Design review of the part built by this model. Coordinates are the model's own, in mm. A direction names the side the tool comes from. Give positions to 0.01 mm unless a question says otherwise; leave off trailing zeros. Write each loop counter-clockwise with the first axis right and the second up, starting at its lowest first coordinate (ties: lowest second). Pieces come first, ordered by that corner, then holes. Notation, with made-up numbers: M 22,54 L 62,54 A13 cw 62,65 Z; hole C 7,-2 d10. An arc over 180 degrees is marked long. Write each question's results on one line, items separated by ' | '. Start each with the question number.
from build123d import *

# Parameters (mm, degrees)
F1_DEPTH = 2
F3_DEPTH = 20
F5_DEPTH = 2


with BuildPart() as f1:
    # F0 (on Top) → F1 (new body)
    with BuildSketch(Plane.XY):
        with BuildLine():
            ThreePointArc((5.3033008589, 5.3033008589), (-6.9290964938, -2.8701257427), (7.5, 0))
            Line((7.5, 0), (5, 0))
            ThreePointArc((5, 0), (-4.6193976626, -1.9134171618), (3.5355339059, 3.5355339059))
            Line((3.5355339059, 3.5355339059), (5.3033008589, 5.3033008589))
        make_face()
        with BuildLine():
            ThreePointArc((3.5355339059, 3.5355339059), (-4.6193976626, -1.9134171618), (5, 0))
            Line((5, 0), (4.6, 0))
            ThreePointArc((4.6, 0), (-4.2498458496, -1.7603437889), (3.2526911935, 3.2526911935))
            Line((3.2526911935, 3.2526911935), (3.5355339059, 3.5355339059))
        make_face()
    extrude(amount=F1_DEPTH)

    # F2 (on face) → F3 (join)
    with BuildSketch(Plane.XY.offset(2)):
        with BuildLine():
            Line((7.5, 0), (5, 0))
            ThreePointArc((5, 0), (-4.6193976626, -1.9134171618), (3.5355339059, 3.5355339059))
            Line((3.5355339059, 3.5355339059), (5.3033008589, 5.3033008589))
            ThreePointArc((5.3033008589, 5.3033008589), (-6.9290964938, -2.8701257427), (7.5, 0))
        make_face()
    extrude(amount=F3_DEPTH)

    # F4 (on face) → F5 (join)
    with BuildSketch(Plane.XY.offset(22)):
        with BuildLine():
            ThreePointArc((3.5355339059, 3.5355339059), (-4.6193976626, -1.9134171618), (5, 0))
            Line((5, 0), (4.6, 0))
            ThreePointArc((4.6, 0), (-4.2498458496, -1.7603437889), (3.2526911935, 3.2526911935))
            Line((3.2526911935, 3.2526911935), (3.5355339059, 3.5355339059))
        make_face()
        with BuildLine():
            ThreePointArc((5.3033008589, 5.3033008589), (-6.9290964938, -2.8701257427), (7.5, 0))
            Line((7.5, 0), (5, 0))
            ThreePointArc((5, 0), (-4.6193976626, -1.9134171618), (3.5355339059, 3.5355339059))
            Line((3.5355339059, 3.5355339059), (5.3033008589, 5.3033008589))
        make_face()
    extrude(amount=F5_DEPTH)


solid = f1.part
Q1. For pin 1 Ø1.5 at (x, z) = (-1, 18) entering from +Y; pin 2 Ø1 at (y, z) = (-3.5, 4.5) entering from +X; pin 3 Ø1.5 at (x, z) = (6, 9) entering from +Y, all flat-tipped, find the tip position at first contact; note any pin that passes through.
Q2. The part is to be moulded in two halves that separate along Z. For faces 1 (the flat face through (-3, -3.7, 2)), 2 (the cylindrical face through (-4.18, -1.92, 0.99)), 3 (the flat face through (-5, 0, 24)), say which applies: pulls with the +Z half, pulls with the -Z half, needs draft (parallel to the pull), parting line crosses it, or undercut.
Q3. We need section A-A on x = 0. Write out the cut boundary in (y, z).
Q4. We need section B-B on y = 4. Write out the cut boundary in (x, z).
Q5. We need section C-C on y = 6. Write out the cut boundary in (x, z).
Q6. We need section D-D on z = 14.75. Write out the cut boundary in (x, y).
Q7. Wall thickness on line 1 along Y through (x, z) = (0, 10); line 2 along Y through (x, z) = (0, 22.8); line 3 along X through (y, z) = (-2.75, 12.5): over which ranges is each line inside the solid? List them lowest first. Write a range as from..to.
Q8. For faces 4 (the cylindrical face through (-4.542, -2.09, 11.86)), 5 (the cylindrical face through (-7.034, -2.601, 11.832)), 6 (the flat face through (6, 0, 12)), list the 3-axis set-ups (+Z, -Z, +X, -X, +Y, -Y) from which the entire face can be reached by the end or side of a thin tool; tool diameter is ignored.
Answer sheet:
1) pin 1: y = 7.5 | pin 2: x = 6.87 | pin 3: y = 5.36
2) face 1: undercut | face 2: needs draft | face 3: pulls with the +Z half
3) outline: M -7.5,0 L -4.6,0 L -4.6,2 L -5,2 L -5,22 L -4.6,22 L -4.6,24 L -7.5,24 Z; M 4.6,0 L 7.5,0 L 7.5,24 L 4.6,24 L 4.6,22 L 5,22 L 5,2 L 4.6,2 Z
4) outline: M -6.34,0 L -2.27,0 L -2.27,2 L -3,2 L -3,22 L -2.27,22 L -2.27,24 L -6.34,24 Z; M 2.27,0 L 4,0 L 4,24 L 2.27,24 L 2.27,22 L 3,22 L 3,2 L 2.27,2 Z
5) outline: M -4.5,0 L 4.5,0 L 4.5,24 L -4.5,24 Z
6) outline: M 3.54,3.54 L 5.3,5.3 A7.5 ccw long 7.5,0 L 5,0 A5 cw long Z
7) line 1: -7.5..-5, 5..7.5 | line 2: -7.5..-4.6, 4.6..7.5 | line 3: -6.98..-4.18, 4.18..6.98
8) face 4: none | face 5: +Z, -Z | face 6: +Z, -Z, +X
